Model file for the job. Use its own axes, mm. A direction names the side the tool comes from. Coordinates: 2 decimals unless noted, no trailing zeros. Order: outer loops, then holes, each group sorted by start corner. A loop starts at its lowest first (then second) coordinate and runs counter-clockwise, first axis right, second up. Notation, with made-up numbers: (23.5, 86.5) -> (41.5, 86.5) arc R23 ccw to (41.5, 112.5) -> close; hole circle Ø8 at (42, -24). An arc over 180 degrees is marked (long way). Write item = value, one per line. Start each with the question number.
Q1. Wall check: line 1 (Y direction, x = -40, z = -2.25); line 2 (Z direction, x = -12, y = 1); line 3 (Y direction, x = -38.5, z = -6.75). Give the ranges that are in metal, low to high. Write a range as from..to.
Q2. Cut at D-D, the plane z = 7.5. List the corners of the cut face in (x, y).
Q3. Cut at A-A, the plane z = -7.5. List the corners of the cut face in (x, y), plus the area to 3 significant figures.
Q4. Flat gauge pins, fed straight in: pin 1 (1 mm diameter, centred on x = -33.5, z = -0.5, fed in from +Y); pin 2 (5 mm diameter, centred on x = 1.5, y = 20, fed in from +Z); pin 3 (5 mm diameter, centred on y = -2, z = 4, fed in from +X); pin 4 (5 mm diameter, centred on x = -34, y = 15, fed in from +Z). Where does each tip first touch, or does it go through?
Q5. Cut at C-C, the plane y = 9.5. List the corners of the cut face in (x, z), plus the area to 3 significant figures.
Q6. 3-axis set-ups, long thin cutter, end or side, ignore diameter. For faces 5 (the face through (-15, 0, 5)), 6 (the face through (0, 0, -5)), 7 (the face through (0, -16, 7)), 8 (the face through (4.5, 19, 7)): which of +Z, -Z, +X, -X, +Y, -Y reach the whole face in a straight line?
Q7. Cut at B-B, the plane y = 2.5. List the corners of the cut face in (x, z).
Q8. Mould opens along X. For faces 1 (the face through (-22.487, 0.778, 2.362)), 2 (the face through (-4.5, 19, 7)), 3 (the face through (0, 19, 4)), 4 (the face through (-32, 0, 0)) say: +X half, -X half, draft (parallel to the pull), parting line (faces both ways), or undercut.
from build123d import *

# Parameters (mm, degrees)
F0_R      = 22.5
F1_DEPTH  = 10
F3_DEPTH  = 20.001
F5_DEPTH  = 6
F7_DEPTH  = 14
F8_W      = 37.5
F8_H      = 10
F9_DEPTH  = 10
F10_W     = 24
F10_H     = 10
F11_DEPTH = 52
F13_DEPTH = 10
F14_D     = 12


with BuildPart() as f1:
    # F0 (on Top) → F1 (new body, symmetric)
    with BuildSketch(Plane.XY):
        Circle(F0_R)
    extrude(amount=F1_DEPTH, both=True)

    # F2 (on face) → F3 (cut, through all)
    with BuildSketch(Plane.XY.offset(10)):
        with BuildLine():
            Line((17.6139149538, 14), (17.6139149538, -14))
            ThreePointArc((17.6139149538, -14), (21.2433882239, -7.4140715379), (22.5, 0))
            ThreePointArc((22.5, 0), (21.2433882239, 7.4140715379), (17.6139149538, 14))
        make_face()
    extrude(amount=-F3_DEPTH, mode=Mode.SUBTRACT)

    # F4 (on face) → F5 (cut)
    with BuildSketch(Plane.XY.offset(10)):
        with BuildLine():
            Line((4.5, -22.045407685), (4.5, -16))
            Line((4.5, -16), (-4.5, -16))
            Line((-4.5, -16), (-4.5, -22.045407685))
            ThreePointArc((-4.5, -22.045407685), (-2.2614516773, -22.3860634394), (-6.48e-08, -22.5))
            ThreePointArc((-6.48e-08, -22.5), (2.2614516129, -22.3860634459), (4.5, -22.045407685))
        make_face()
        with BuildLine():
            ThreePointArc((4.5, 22.045407685), (2.2614515402, 22.3860634532), (-2.11e-07, 22.5))
            ThreePointArc((-2.11e-07, 22.5), (-2.2614517501, 22.386063432), (-4.5, 22.045407685))
            Line((-4.5, 22.045407685), (-4.5, 16))
            Line((-4.5, 16), (4.5, 16))
            Line((4.5, 16), (4.5, 22.045407685))
        make_face()
    extrude(amount=-F5_DEPTH, mode=Mode.SUBTRACT)

    # F6 (on Front) → F7 (cut, symmetric)
    with BuildSketch(Plane.XZ):
        Polygon((17.6139149538, 3), (17.6139149538, 10), (0, 10), align=None)
    extrude(amount=F7_DEPTH, both=True, mode=Mode.SUBTRACT)

    # F8 (on Top) → F9 (cut, symmetric)
    with BuildSketch(Plane.XY):
        with Locations((3.75, 0)):
            Rectangle(F8_W, F8_H)
    extrude(amount=F9_DEPTH, both=True, mode=Mode.SUBTRACT)

    # F10 (on Right) → F11 (join)
    with BuildSketch(Plane.YZ):
        with Locations((0, -5)):
            Rectangle(F10_W, F10_H)
    extrude(amount=-F11_DEPTH)

    # F12 (on Top) → F13 (cut)
    with BuildSketch(Plane.XY):
        with BuildLine():
            Line((-40, 12), (-52, 12))
            Line((-52, 12), (-52, 0))
            ThreePointArc((-52, 0), (-48.4852813742, 8.4852813742), (-40, 12))
        make_face()
        with BuildLine():
            ThreePointArc((-40, -12), (-48.4852813742, -8.4852813742), (-52, 0))
            Line((-52, 0), (-52, -12))
            Line((-52, -12), (-40, -12))
        make_face()
    extrude(amount=-F13_DEPTH, mode=Mode.SUBTRACT)

    # F14 (through all)
    with Locations(Plane.XY):
        with Locations((-40, 0)):
            Hole(F14_D / 2)


solid = f1.part
Here are the results:
q1.line_1 = -12..-6, 6..12
q1.line_2 = -10..0
q1.line_3 = -12..-5.81, 5.81..12
q2.outline = (-15, -5) -> (-15, 5) -> (6.29, 5) -> (6.29, 14) -> (17.61, 14) arc R22.5 ccw to (4.5, 22.05) -> (4.5, 16) -> (-4.5, 16) -> (-4.5, 22.05) arc R22.5 ccw to (-4.5, -22.05) -> (-4.5, -16) -> (4.5, -16) -> (4.5, -22.05) arc R22.5 ccw to (17.61, -14) -> (6.29, -14) -> (6.29, -5) -> close
q3.outline = (-40, -12) -> (-19.03, -12) arc R22.5 ccw to (17.61, -14) -> (17.61, -5) -> (0, -5) -> (0, 5) -> (17.61, 5) -> (17.61, 14) arc R22.5 ccw to (-19.03, 12) -> (-40, 12) arc R12 ccw to start; hole circle Ø12 at (-40, 0)
q3.area = 1,880 mm²
q4.pin_1 = 12
q4.pin_2 = 4
q4.pin_3 = -15
q4.pin_4 = through
q5.outline = (-47.33, -10) -> (17.61, -10) -> (17.61, 3) -> (0, 10) -> (-20.4, 10) -> (-20.4, 0) -> (-47.33, 0) -> close
q5.area = 968 mm²
q6.face_5 = +Z, +X
q6.face_6 = +Z, -Z, +X
q6.face_7 = +Z, -Y
q6.face_8 = +Z, +Y
q7.outline = (-51.74, -10) -> (-45.45, -10) -> (-45.45, 0) -> (-51.74, 0) -> close; (-34.55, -10) -> (0, -10) -> (0, 0) -> (-15, 0) -> (-15, 10) -> (-22.36, 10) -> (-22.36, 0) -> (-34.55, 0) -> close
q8.face_1 = parting line
q8.face_2 = undercut
q8.face_3 = undercut
q8.face_4 = draft
